Autodesk Inventor part; units mm, degrees
ref_plane "Work Plane1" through (0, 0, 100) normal (0, 0, 1) x (1, 0, 0)
ref_plane "YZ Plane" through (0, 0, 0) normal (1, 0, 0) x (0, 1, 0)
ref_plane "XZ Plane" through (0, 0, 0) normal (0, 1, 0) x (-1, 0, 0)
sketch "Sketch3" plane through (0, 0, 0) normal (0, 1, 0) x (-1, 0, 0)
  line L0 (0, 0) -> (0, 31.5556)
sketch "Sketch1" plane through (0, 0, 0) normal (0, 0, 1) x (1, 0, 0)
  circle A0 centre (0, 0) radius 75
  circle A1 centre (63.483, 20.6269) radius 6 construction
  circle A2 centre (-63.483, -20.6269) radius 6 construction
  circle A3 centre (0, 0) radius 69 construction
  line L0 (0, 0) -> (0.0001, -211.0949) construction
  arc A4 (-59.7327, 15.2299) -> (-60.2661, -15.5622) centre (-48.002, -0.374) ccw construction
  line L1 (0.2505, 0.4177) -> (-45.224, -139.5383) construction
  line L2 (-0.1358, 0.4177) -> (49.2707, -151.6398) construction
  line L3 (0, 0) -> (0.0001, -82)
  line L4 (0.0001, -82) -> (0.0001, -112)
  circle A5 centre (0.0001, -82) radius 2
  circle A6 centre (0.0001, -112) radius 2
  line L5 (0.0001, -82) -> (25.0001, -82)
  line L6 (0.0001, -82) -> (-24.9999, -82)
  line L7 (25.0001, -112) -> (25.0001, -70.7106)
  line L8 (-24.9999, -112) -> (-24.9999, -70.7107)
  line L9 (25.0001, -125) -> (25.0001, -112)
  line L10 (25.0001, -125) -> (-24.9999, -125)
  line L11 (-24.9999, -125) -> (-24.9999, -112)
  point P0 (56.6452, 18.2098)
  point P1 (56.6452, 18.2098)
  point P2 (57.7767, 18.7728)
  point P3 (56.6452, 18.2098)
  point P4 (57.7767, 18.7728)
  point P5 (56.6794, 18.5913)
  point P6 (-19.8743, -61.5198)
  point P7 (19.9889, -61.5198)
  point P8 (19.9889, -61.5198)
  point P9 (0.0001, -75)
  dimension "d19" = 12
  dimension "d66" = 12
  dimension "d4" = 150
  dimension "d59" = 66.75
  dimension "d67" = 63.483
  dimension "d68" = 138
  dimension "d147" = 18
  dimension "d148" = 18
  dimension "d157" = 82
  dimension "d158" = 30
  dimension "d159" = 4
  dimension "d160" = 4
  dimension "d161" = 25
  dimension "d162" = 25
  dimension "d163" = 25
  dimension "d164" = 25
  dimension "d165" = 50
ref_plane "Work Plane1" through (0, 0, 100) normal (0, 0, 1) x (1, 0, 0)
sketch "Sketch9" plane through (0, 0, 100) normal (0, 0, 1) x (1, 0, 0)
  circle A0 centre (0, 0) radius 75
  spline S0 degree 3 number of poles 235
  circle A1 centre (0, 0) radius 69
  line L0 (0, -270.1399) -> (0, 140.0417) construction
  line L1 (-118.2892, 0) -> (124.185, 0) construction
  point P0 (0, 0)
  point P1 (59.5, 0)
  point P2 (69, 0)
  dimension "d112" = 69
extrude "Extrusion7" [suppressed]
sketch "Sketch10" plane through (0, 0, 2.5) normal (0, 0, 1) x (1, 0, 0)
  circle A0 centre (69, 0) radius 1.5
  line L0 (71.75, -1.5877) -> (69, -3.1754)
  line L1 (69, -3.1754) -> (66.25, -1.5877)
  line L2 (66.25, -1.5877) -> (66.25, 1.5877)
  line L3 (66.25, 1.5877) -> (69, 3.1754)
  line L4 (69, 3.1754) -> (71.75, 1.5877)
  line L5 (71.75, 1.5877) -> (71.75, -1.5877)
  point P0 (0, 0)
  dimension "d115" = 3
  dimension "d118" = 5.5
extrude "Extrusion10" [suppressed]
pattern_circular "Circular Pattern4" [suppressed]
extrude "Extrusion8" [suppressed]
extrude "Extrusion9" [suppressed]
pattern_circular "Circular Pattern3" [suppressed]
extrude "Extrusion3" [suppressed]
sketch "Sketch12" plane through (0, 0, -13.15) normal (0, 0, -1) x (-1, 0, 0)
  circle A0 centre (0, 0) radius 69
  point P0 (-65.6229, -21.3222)
  dimension "d132" = 138
hole "Hole3" [suppressed]
pattern_circular "Circular Pattern5" [suppressed]
sketch "Sketch13" plane through (0, 0, 0) normal (0, 1, 0) x (-1, 0, 0)
  line L0 (-64.5572, 13.15) -> (64.4426, 13.15)
  line L1 (-64.5572, -13.15) -> (64.4426, -13.15)
  line L2 (75, 13.15) -> (-75, 13.15)
  line L3 (-23.4889, 2.0207) -> (-19.9889, 4.0415)
  line L4 (-19.9889, 4.0415) -> (-16.4889, 2.0207)
  line L5 (-16.4889, 2.0207) -> (-16.4889, -2.0207)
  line L6 (-16.4889, -2.0207) -> (-19.9889, -4.0415)
  line L7 (-19.9889, -4.0415) -> (-23.4889, -2.0207)
  line L8 (-23.4889, -2.0207) -> (-23.4889, 2.0207)
  line L9 (16.3743, 2.0207) -> (19.8743, 4.0415)
  line L10 (19.8743, 4.0415) -> (23.3743, 2.0207)
  line L11 (23.3743, 2.0207) -> (23.3743, -2.0207)
  line L12 (23.3743, -2.0207) -> (19.8743, -4.0415)
  line L13 (19.8743, -4.0415) -> (16.3743, -2.0207)
  line L14 (16.3743, -2.0207) -> (16.3743, 2.0207)
  circle A0 centre (19.8743, 0) radius 2
  circle A1 centre (-19.9889, 0) radius 2
  point P0 (0, 0)
  point P1 (-56.6452, 13.15)
  point P2 (-56.6452, -13.15)
  dimension "d149" = 7
  dimension "d150" = 7
  dimension "d153" = 4
  dimension "d154" = 4
extrude "Extrusion12" [suppressed]
extrude "Extrusion13" [suppressed]
extrude "Extrusion14" add sketch "Sketch1" along normal mid plane 26.3 contours A0 L3 A5 L6 L8 | L7 L5 A5 L3 A0 | L6 A5 L5 L7 L9 L10 L11 L8
sketch "Sketch14" plane through (-24.9999, -125, 13.15) normal (0, -1, 0) x (1, 0, 0)
  circle A0 centre (5.1257, -13.15) radius 2
  line L0 (8.6257, -11.1293) -> (5.1257, -9.1085)
  line L1 (5.1257, -9.1085) -> (1.6257, -11.1293)
  line L2 (1.6257, -11.1293) -> (1.6257, -15.1707)
  line L3 (1.6257, -15.1707) -> (5.1257, -17.1915)
  line L4 (5.1257, -17.1915) -> (8.6257, -15.1707)
  line L5 (8.6257, -15.1707) -> (8.6257, -11.1293)
  line L6 (44.9889, -9.1085) -> (41.4889, -11.1293)
  circle A1 centre (44.9889, -13.15) radius 2
  line L7 (48.4889, -11.1293) -> (44.9889, -9.1085)
  line L8 (48.4889, -15.1707) -> (48.4889, -11.1293)
  line L9 (44.9889, -17.1915) -> (48.4889, -15.1707)
  line L10 (41.4889, -15.1707) -> (44.9889, -17.1915)
  line L11 (41.4889, -11.1293) -> (41.4889, -15.1707)
  point P0 (24.9999, -13.15)
extrude "Extrusion15" cut sketch "Sketch14" against normal through all contours A0 | A1
extrude "Extrusion16" cut sketch "Sketch14" against normal blind 4 contours A0 | L5 L4 L3 L2 L1 L0 | L7 L8 L9 L10 L11 L6 | A1
sketch "Sketch15" plane through (0, 0, 13.15) normal (0, 0, 1) x (1, 0, 0)
  line L0 (-24.9999, -70.7107) -> (-24.9999, -125)
  line L1 (-24.9999, -125) -> (25.0001, -125)
  line L2 (25.0001, -125) -> (25.0001, -70.7106)
  arc A0 (-24.9999, -70.7107) -> (25.0001, -70.7106) centre (0, 0) ccw
  circle A1 centre (0.0001, -82) radius 2
  circle A2 centre (0.0001, -112) radius 2
  point P0 (0, 0)
  dimension "d99" = 156
extrude "Extrusion17" add sketch "Sketch15" along normal blind 32.694
fillet "Fillet2" radius 8 3 edges at (25.0001, -97.8553, 45.844) (-24.9999, -97.8554, 45.844) (0.0001, -125, 45.844)
sketch "Sketch8" plane through (0, 0, -13.15) normal (0, 0, -1) x (-1, 0, 0)
  circle A0 centre (0, 0) radius 78
  arc A1 (-23.65, -105.9607) -> (-46.4722, -58.8671) centre (-83.65, -105.9607) ccw
  arc A2 (46.4722, -58.8671) -> (23.65, -105.9607) centre (83.65, -105.9607) ccw
  line L0 (23.65, -200) -> (23.65, -105.9607)
  line L1 (-23.65, -105.9607) -> (-23.65, -200)
  arc A3 (-23.65, -200) -> (23.65, -200) centre (0, -181.5425) ccw
  point P0 (36.3948, -68.9886)
  point P1 (-36.3948, -68.9886)
sketch "Sketch11" plane through (0, 0, 2.5) normal (0, 0, 1) x (1, 0, 0)
  circle A0 centre (0, 0) radius 11.25
  dimension "d129" = 22.5
equation "\"Axle_diameter\" = 6"
equation "\"Compensation\" = 0.45"
equation "\"Bearing_Outer_Hole_Location\" = 138"
equation "\"Printer_Gap_Fit\" = 0.1"
equation "\"Printer_Gap_Slide\" = 0.3"
equation "\"Bearing_Roller_Diameter\" = 8"
equation "\"Fastners_ScrewHeadThickness\" = 2"
equation "\"Fastners_OuterThicknessFromScrew\" = 5"
equation "\"Fastners_InnerThicknessFromScrew\" = 2"
equation "\"Fastners_OutputAxisHeadThickness\" = 2"
equation "\"Printer_HoleCompensation\" = 0"
equation "\"Bearing_Outer_Radius\" = 75"
equation "\"Bearing_Thicness_compensation\" = 0.27244"
equation "\"Bearing_To_12mm\" = 0.27244"
equation "\"Bearing_Inner_Hole_Location\" = 84"
equation "\"Housing_Outer_Hole_Location\" = 138"
equation "\"Bearing_Gap_Fit\" = 0.1"
equation "\"Bearing_Gap_Slide\" = 0.43"
equation "\"Bearing_ScrewHeadThickness\" = 2"
equation "\"Bearing_OuterThicknessFromScrew\" = 5"
equation "\"Bearing_InnerThicknessFromScrew\" = 2"
equation "\"Bearing_OutputAxisHeadThickness\" = 2"
equation "\"Bearing_HoleCompensation\" = 0.5"
equation "\"Roller_radius\" = 5"
equation "\"Pin_set_dimention\" = 22"
equation "\"Pin_bearing_outer_dimention\" = 22"
equation "\"Shaft_dimention\" = 2"
equation "\"Pin_bearing_inner_dimention\" = 3"
equation "\"Rotor_dimention\" = 125"
equation "\"Rotor_radius\" = 62.5"
equation "\"Outer_rotor_radius\" = 65"
equation "\"Output_hole_set_diameter\" = 24.5"
equation "\"Bearing_ScrewDiameter\" = 3.5"
equation "\"Bearing_ScrewHeadDiameter\" = 5.5"
equation "\"Bearing_OutputAxisHeadDiameter\" = 8.5"
equation "\"BearingHoleThrough\" = 12"
equation "\"Fastners_ScrewDiameter\" = 3"
equation "\"Bearing_OutputAxisDiameter\" = 6"
equation "\"Fastners_ScrewHeadDiameter\" = 5"
equation "\"Fastners_OutputAxisHeadDiameter\" = 12"
equation "\"BraceMountThickness\" = 47.3"
equation "\"R\" = 1"
equation "\"Rr\" = 1"
equation "\"Ece\" = 1"
equation "\"Num\" = 1"
equation "\"formula\" = 1"
properties part number "AttatchmentUpper" material "ABS Plastic"
The model under review builds one solid part; all positions refer to its coordinate system, in mm. A direction names the side the tool comes from. Give positions to 0.01 mm unless a question says otherwise; leave off trailing zeros. Write each loop counter-clockwise with the first axis right and the second up, starting at its lowest first coordinate (ties: lowest second). Pieces come first, ordered by that corner, then holes. Notation, with made-up numbers: M 16.25,17 L 26.25,17 A26 ccw 26.25,36 Z; hole C 17.25,74.5 d7. An arc over 180 degrees is marked long. Write each question's results on one line, items separated by ' | '. Start each with the question number.
1. We need section B-B (z = 0). Write out the cut boundary in (x, y).
2. We need section C-C (y = -99.5). Write out the cut boundary in (x, z).
3. Mouldability with a two-part tool opening along Y and no side actions: class faces 3 (the flat face through (-16.374, -123, 0)), 4 (the cylindrical face through (0, -75, 0)), 5 (the cylindrical face through (0, -84, 16)) as released by +Y, released by -Y, zero draft, split by the parting line, or undercut.
4. We need section D-D (z = 35). Write out the cut boundary in (x, y).
5. For faces 1 (the cylindrical face through (21.836, -96.697, -0.766)), 2 (the flat face through (-21, -121, -2)), list the 3-axis set-ups (+Z, -Z, +X, -X, +Y, -Y) from which the entire face can be reached by the end or side of a thin tool; tool diameter is ignored.
6. Insertion check: pin 1 Ø4 at (x, z) = (-10.5, -4.5) entering from +Y; pin 2 Ø3.5 at (x, z) = (18.5, 0.5) entering from -Y; pin 3 Ø8 at (x, z) = (-19, 23.5) entering from +Y; pin 4 Ø2.5 at (x, z) = (19.989, 0) entering from -Y. Each pin has a flat end and moves straight along its axis. Give the tip position at first contact, or say it passes through.
7. We need section A-A (y = -112). Write out the cut boundary in (x, z), and give its area (3 significant figures).
8. For probe 1 along X at (y, z) = (-101, 0); probe 2 along Y at (x, z) = (1.5, 5) (3 decimals); probe 3 along Y at (x, z) = (-1, 18), list the stretches that pass through material, from the lowest coordinate up. Write a range as [from, to].
Results found:
1) outline: M -25,-125 L -23.37,-125 L -23.37,-121 L -21.87,-121 L -21.87,-71.74 A75 cw -25,-70.71 Z; M -17.87,-121 L -16.37,-121 L -16.37,-125 L 16.49,-125 L 16.49,-121 L 17.99,-121 L 17.99,-72.81 A75 cw -17.87,-72.84 Z; M 21.99,-121 L 23.49,-121 L 23.49,-125 L 25,-125 L 25,-70.71 A75 cw 21.99,-71.7 Z; hole C 0,-112 d4; hole C 0,-82 d4
2) outline: M -25,-13.15 L 25,-13.15 L 25,37.84 A8 ccw 17,45.84 L -17,45.84 A8 ccw -25,37.84 Z; hole C -19.87,0 d4; hole C 19.99,0 d4
3) face 3: zero draft | face 4: released by +Y | face 5: undercut
4) outline: M -25,-125 L 25,-125 L 25,-70.71 A75 cw -25,-70.71 Z; hole C 0,-112 d4; hole C 0,-82 d4
5) face 1: +Y, -Y | face 2: -Y
6) pin 1: stops at y = -73.95 | pin 2: stops at y = -121 | pin 3: stops at y = -71.39 | pin 4: passes through
7) outline: M -25,-13.15 L -2,-13.15 L -2,45.84 L -17,45.84 A8 ccw -25,37.84 Z; M 2,-13.15 L 25,-13.15 L 25,37.84 A8 ccw 17,45.84 L 2,45.84 Z; hole C -19.87,0 d4; hole C 19.99,0 d4 | area: 2,660 mm^2
8) probe 1: x = [-25, -21.87], [-17.87, 17.99], [21.99, 25] | probe 2: y = [-125, -113.323], [-110.677, -83.323], [-80.677, -74.985] | probe 3: y = [-125, -113.73], [-110.27, -83.73], [-80.27, -74.99]
